from build123d import *

# Parameters (mm, degrees)
SKETCH1_R           = 11.049
BOSS_EXTRUDE1_DEPTH = 1.5875
SKETCH2_R           = 8.0899
BOSS_EXTRUDE2_DEPTH = 12.7
SKETCH3_R           = 11.049
BOSS_EXTRUDE3_DEPTH = 1.5875
SKETCH4_R           = 6.35
BOSS_EXTRUDE4_DEPTH = 6.35
SKETCH5_R           = 2.38125
CUT_EXTRUDE1_DEPTH  = 25.4


with BuildPart() as part:
    # Sketch1 → Boss-Extrude1 (new body)
    with BuildSketch(Plane.XY):
        Circle(SKETCH1_R)
    extrude(amount=BOSS_EXTRUDE1_DEPTH)

    # Sketch2 → Boss-Extrude2 (add)
    with BuildSketch(Plane.XY.offset(1.5875)):
        Circle(SKETCH2_R)
    extrude(amount=BOSS_EXTRUDE2_DEPTH)

    # Sketch3 → Boss-Extrude3 (add)
    with BuildSketch(Plane.XY.offset(14.2875)):
        Circle(SKETCH3_R)
    extrude(amount=BOSS_EXTRUDE3_DEPTH)

    # Sketch4 → Boss-Extrude4 (add)
    with BuildSketch(Plane.XY.offset(15.875)):
        Circle(SKETCH4_R)
    extrude(amount=BOSS_EXTRUDE4_DEPTH)

    # Sketch5 → Cut-Extrude1 (cut)
    with BuildSketch(Plane.XY.offset(22.225)):
        Circle(SKETCH5_R)
    extrude(amount=-CUT_EXTRUDE1_DEPTH, mode=Mode.SUBTRACT)


solid = part.part
Here's how the part is built. I have some questions about the finished solid (model axes, mm). A direction names the side the tool comes from. Round coordinates to 2 decimals unless told otherwise and drop trailing zeros. Order: outer loops, then holes, each group sorted by start corner. A loop starts at its lowest first (then second) coordinate and runs counter-clockwise, first axis right, second up. Notation, with made-up numbers: M 17,-24 L 42,-24 A35 cw 42,11 Z; hole C 8,89.25 d3. An arc over 180 degrees is marked long. Return JSON: item names as keys, results as strings. Group by question number.
1. Please list where these lines run through material, in increasing order: probe 1 along Z at (x, y) = (-10, -0.5) (1 decimal); probe 2 along Y at (x, z) = (0, 8.5); probe 3 along Y at (x, z) = (0, 15.75).
2. If we section it at D-D on x = -9.5: List the corners of the cut face in (y, z) for me (1 decimal).
3. On a 3-axis mill with a long thin cutter (end or side, diameter ignored), from which of +Z, -Z, +X, -X, +Y, -Y can I reach the whole of each face in a straight line? I mean faces 5 (the face through (-6, 6, 14.288)), 6 (the face through (-1.89, -1.45, 11.27)). Say none if no direction works.
4. If we section it at C-C on z = 4.75: List the corners of the cut face in (x, y) for me.
5. If we mould it in two halves opening along Z, with no side actions, what happens to faces 1 (the face through (5, -5, 15.875)), 2 (the face through (7.716, 2.43, 7.849)), 3 (the face through (-6, 6, 1.588)), 4 (the face through (-1.38, -6.2, 19.01))? For each: pulls with the +Z half, pulls with the -Z half, needs draft (parallel to the pull), parting line crosses it, or undercut.
6. I'm going to push flat-ended pins straight in: pin 1 Ø1.5 at (x, z) = (0.5, 11.5) entering from -Y; pin 2 Ø4 at (x, y) = (4, 7.5) entering from +Z (3 decimals); pin 3 Ø3 at (y, z) = (8.5, 10.5) entering from -X; pin 4 Ø4.5 at (x, y) = (0, 0) entering from +Z. Where does each tip first touch, or does it pass through?
Reply:
{
 "1": {"probe 1": "0 to 1.6, 14.3 to 15.9", "probe 2": "-8.09 to -2.38, 2.38 to 8.09", "probe 3": "-11.05 to -2.38, 2.38 to 11.05"},
 "2": {"outline": "M -5.6,0 L 5.6,0 L 5.6,1.6 L -5.6,1.6 Z; M -5.6,14.3 L 5.6,14.3 L 5.6,15.9 L -5.6,15.9 Z"},
 "3": {"face 5": "none", "face 6": "+Z, -Z"},
 "4": {"outline": "C 0,0 d16.18; hole C 0,0 d4.76"},
 "5": {"face 1": "pulls with the +Z half", "face 2": "undercut", "face 3": "undercut", "face 4": "needs draft"},
 "6": {"pin 1": "y = -8.09", "pin 2": "z = 15.875", "pin 3": "x = -4.06", "pin 4": "through"}
}
